Job drawing, mm, ordinate dimensions from the low corner. One solid piece. Coordinates: 2 decimals unless noted, no trailing zeros. Loops run counter-clockwise (first coordinate to the right, second up) from the corner with the lowest first, then second, coordinate; pieces in that order, holes last. Notation, with made-up numbers: (7, 28.5) -> (47, 28.5) arc R15 ccw to (47, 53.5) -> close; hole circle Ø5 at (-18.5, -9.5). An arc over 180 degrees is marked (long way). Answer as CSV lines item,"result". Start each with the question number.
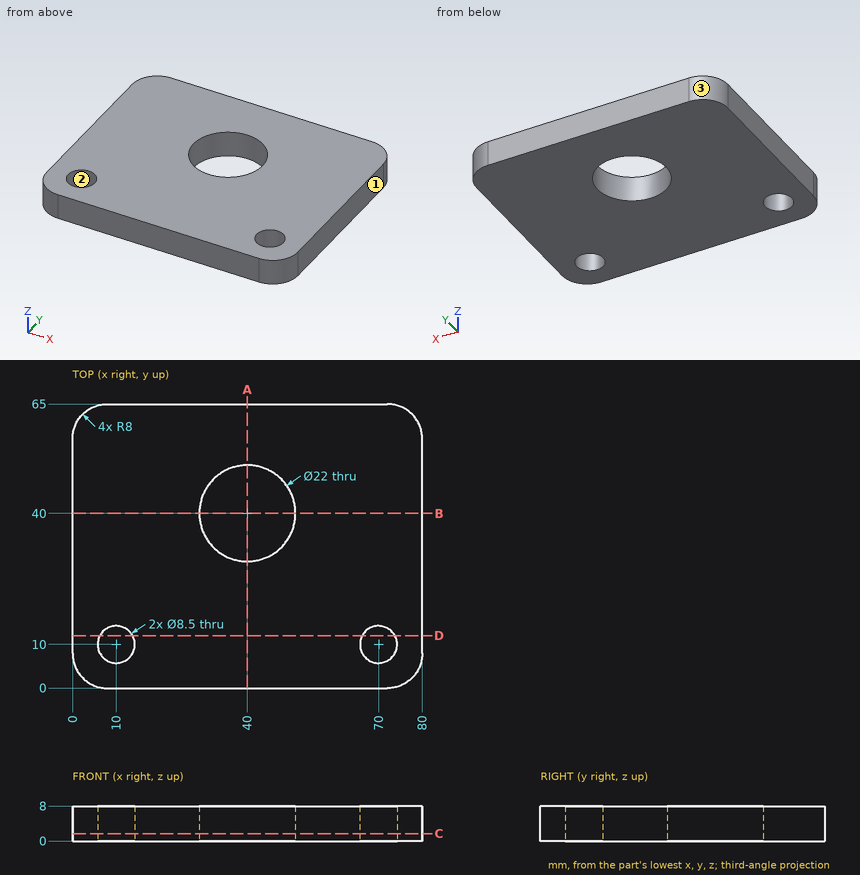
Q1. Pin check, flat tip, straight feed: pin 1 Ø7.5 at (x, y) = (70, 10) entering from -Z. Stop position of the tip, or through.
Q2. Saw through at C-C (z = 1.75). List the corners of the cut face in (x, y), and give its area (3 significant figures).
Q3. Two-plate mould, pull along X, no slides. Class the marked faces 1, 2 and 3: pulls with the +X half, pulls with the -X half, needs draft (parallel to the pull), parting line crosses it, or undercut.
Q4. Saw through at D-D (y = 12). List the corners of the cut face in (x, z).
Q5. Probe probe 1 along Y at (x, z) = (40, 5.75); probe 2 along Y at (x, z) = (70, 5.25); probe 3 along X at (y, z) = (10.5, 1.5). List the from-to ranges inside material, lowest first. Write a range as from..to.
Q6. Saw through at A-A (x = 40). List the corners of the cut face in (y, z), and give its area (3 significant figures).
Q7. Saw through at B-B (y = 40). List the corners of the cut face in (x, z), and give its area (3 significant figures).
Ans:
1,pin 1,"passes through"
2,outline,"(0, 8) arc R8 ccw to (8, 0) -> (72, 0) arc R8 ccw to (80, 8) -> (80, 57) arc R8 ccw to (72, 65) -> (8, 65) arc R8 ccw to (0, 57) -> close; hole circle Ø8.5 at (10, 10); hole circle Ø22 at (40, 40); hole circle Ø8.5 at (70, 10)"
2,area,"4,650 mm²"
3,face 1,"pulls with the +X half"
3,face 2,"undercut"
3,face 3,"pulls with the -X half"
4,outline,"(0, 0) -> (6.25, 0) -> (6.25, 8) -> (0, 8) -> close; (13.75, 0) -> (66.25, 0) -> (66.25, 8) -> (13.75, 8) -> close; (73.75, 0) -> (80, 0) -> (80, 8) -> (73.75, 8) -> close"
5,probe 1,"y = 0..29, 51..65"
5,probe 2,"y = 0..5.75, 14.25..65"
5,probe 3,"x = 0..5.78, 14.22..65.78, 74.22..80"
6,outline,"(0, 0) -> (29, 0) -> (29, 8) -> (0, 8) -> close; (51, 0) -> (65, 0) -> (65, 8) -> (51, 8) -> close"
6,area,"344 mm²"
7,outline,"(0, 0) -> (29, 0) -> (29, 8) -> (0, 8) -> close; (51, 0) -> (80, 0) -> (80, 8) -> (51, 8) -> close"
7,area,"464 mm²"
